Work out the finished part from the listing and answer in its coordinate system (mm). A direction names the side the tool comes from. Coordinates: 2 decimals unless noted, no trailing zeros. Order: outer loops, then holes, each group sorted by start corner. A loop starts at its lowest first (then second) coordinate and runs counter-clockwise, first axis right, second up. Notation, with made-up numbers: M 19.25,10.5 L 46.25,10.5 A21 cw 46.25,48.5 Z; hole C -12.75,78.5 d7. An arc over 180 degrees is marked long. Use a Markdown table: item, result. Add a question column.
from build123d import *

# Parameters (mm, degrees)
BOSS_EXTRUDE1_DEPTH      = 9.525
BOSS_EXTRUDE1_DEPTH_BACK = 9.525
SKETCH1_R                = 1.7
CUT_EXTRUDE1_DEPTH       = 6.35
CUT_EXTRUDE1_DEPTH_BACK  = 27.686
SKETCH2_W                = 2.54
SKETCH2_H                = 5.08
BOSS_EXTRUDE2_DEPTH      = 1.5875
BOSS_EXTRUDE3_START      = 1.5875
SKETCH5_R                = 1.7
BOSS_EXTRUDE3_DEPTH      = 1.5875
CUT_EXTRUDE2_START       = -5.08
CUT_EXTRUDE2_DEPTH       = 5.08
FILLET1_R                = 6.35
FILLET2_R                = 2.54
CHAMFER1_SIZE            = 0.5
SKETCH8_W                = 17.78
SKETCH8_H                = 50.8
CUT_EXTRUDE3_DEPTH       = 5.08
FILLET3_START            = -0.635
FILLET3_DEPTH            = 5.635


with BuildPart() as part:
    # Sketch1 → Boss-Extrude1 (new, two sides: drawn at the far end of the back side and taken through both)
    with BuildSketch(Plane.XY.offset(-BOSS_EXTRUDE1_DEPTH_BACK)):
        with BuildLine():
            Line((-107.95, 0), (-133.35, 0))
            Line((-133.35, 0), (-133.35, -17.78))
            Line((-133.35, -17.78), (-123.825, -17.78))
            ThreePointArc((-123.825, -17.78), (-117.475, -11.43), (-111.125, -17.78))
            Line((-111.125, -17.78), (-101.7905, -17.78))
            Line((-101.7905, -17.78), (-101.7905, -3.81))
            ThreePointArc((-101.7905, -3.81), (-100.302602448, -0.217897552), (-96.7105, 1.27))
            Line((-96.7105, 1.27), (-93.9165, 1.27))
            ThreePointArc((-93.9165, 1.27), (-90.324397552, -0.217897552), (-88.8365, -3.81))
            Line((-88.8365, -3.81), (-88.8365, -17.78))
            Line((-88.8365, -17.78), (-88.8365, -33.02))
            Line((-88.8365, -33.02), (88.8365, -33.02))
            Line((88.8365, -33.02), (88.8365, -17.78))
            Line((88.8365, -17.78), (88.8365, -3.81))
            ThreePointArc((88.8365, -3.81), (90.324397552, -0.217897552), (93.9165, 1.27))
            Line((93.9165, 1.27), (96.7105, 1.27))
            ThreePointArc((96.7105, 1.27), (100.302602448, -0.217897552), (101.7905, -3.81))
            Line((101.7905, -3.81), (101.7905, -17.78))
            Line((101.7905, -17.78), (111.125, -17.78))
            ThreePointArc((111.125, -17.78), (117.475, -11.43), (123.825, -17.78))
            Line((123.825, -17.78), (133.35, -17.78))
            Line((133.35, -17.78), (133.35, 0))
            Line((133.35, 0), (107.95, 0))
            Line((107.95, 0), (107.95, 17.78))
            Line((107.95, 17.78), (-107.95, 17.78))
            Line((-107.95, 17.78), (-107.95, 0))
        make_face()
        with Locations((-79.9465, -7.62)):
            Circle(SKETCH1_R, mode=Mode.SUBTRACT)
        with Locations((-79.9465, 11.43)):
            Circle(SKETCH1_R, mode=Mode.SUBTRACT)
        with Locations((79.9465, -7.62)):
            Circle(SKETCH1_R, mode=Mode.SUBTRACT)
        with Locations((79.9465, 11.43)):
            Circle(SKETCH1_R, mode=Mode.SUBTRACT)
    extrude(amount=BOSS_EXTRUDE1_DEPTH + BOSS_EXTRUDE1_DEPTH_BACK)

    # Sketch2 → Cut-Extrude1 (cut, two sides: drawn at the far end of the back side and taken through both)
    with BuildSketch(Plane(origin=(0, 0, 0), x_dir=(1, 0, 0), z_dir=(0, 1, 0)).offset(-CUT_EXTRUDE1_DEPTH_BACK)):
        with Locations((-106.68, 0)):
            Rectangle(SKETCH2_W, SKETCH2_H)
        with Locations((-132.08, 0)):
            Rectangle(SKETCH2_W, SKETCH2_H)
        with Locations((132.08, 0)):
            Rectangle(SKETCH2_W, SKETCH2_H)
        with Locations((106.68, 0)):
            Rectangle(SKETCH2_W, SKETCH2_H)
    extrude(amount=CUT_EXTRUDE1_DEPTH + CUT_EXTRUDE1_DEPTH_BACK, mode=Mode.SUBTRACT)

    # Sketch3 → Boss-Extrude2 (add)
    with BuildSketch(Plane.XY.offset(9.525)):
        with BuildLine():
            Line((-101.7905, -17.78), (-101.7905, 0))
            Line((-101.7905, 0), (-133.35, 0))
            Line((-133.35, 0), (-133.35, -17.78))
            Line((-133.35, -17.78), (-122.301, -17.78))
            ThreePointArc((-122.301, -17.78), (-117.475, -12.954), (-112.649, -17.78))
            Line((-112.649, -17.78), (-101.7905, -17.78))
        make_face()
        with BuildLine():
            Line((101.7905, -17.78), (112.649, -17.78))
            ThreePointArc((112.649, -17.78), (117.475, -12.954), (122.301, -17.78))
            Line((122.301, -17.78), (133.35, -17.78))
            Line((133.35, -17.78), (133.35, 0))
            Line((133.35, 0), (101.7905, 0))
            Line((101.7905, 0), (101.7905, -17.78))
        make_face()
    boss_extrude2 = extrude(amount=BOSS_EXTRUDE2_DEPTH)

    # Mirror1: Boss-Extrude2 across plane
    add(boss_extrude2.mirror(Plane.XY))

    # Sketch5 → Boss-Extrude3 (add)
    with BuildSketch(Plane(origin=(0, 0, -9.525), x_dir=(-1, 0, 0), z_dir=(0, 0, -1)).offset(BOSS_EXTRUDE3_START)):
        with BuildLine():
            Line((-107.95, 0), (-101.7905, 0))
            Line((-101.7905, 0), (-101.7905, -3.81))
            ThreePointArc((-101.7905, -3.81), (-100.302602448, -0.217897552), (-96.7105, 1.27))
            Line((-96.7105, 1.27), (-93.9165, 1.27))
            ThreePointArc((-93.9165, 1.27), (-90.324397552, -0.217897552), (-88.8365, -3.81))
            Line((-88.8365, -3.81), (-88.8365, -33.02))
            Line((-88.8365, -33.02), (88.8365, -33.02))
            Line((88.8365, -33.02), (88.8365, -3.81))
            ThreePointArc((88.8365, -3.81), (90.324397552, -0.217897552), (93.9165, 1.27))
            Line((93.9165, 1.27), (96.7105, 1.27))
            ThreePointArc((96.7105, 1.27), (100.302602448, -0.217897552), (101.7905, -3.81))
            Line((101.7905, -3.81), (101.7905, 0))
            Line((101.7905, 0), (107.95, 0))
            Line((107.95, 0), (107.95, 17.78))
            Line((107.95, 17.78), (-107.95, 17.78))
            Line((-107.95, 17.78), (-107.95, 0))
        make_face()
        with Locations(Location((-79.9465, -7.62, 0), (0, 0, 180))):
            Circle(SKETCH5_R, mode=Mode.SUBTRACT)
        with Locations(Location((-79.9465, 11.43, 0), (0, 0, 180))):
            Circle(SKETCH5_R, mode=Mode.SUBTRACT)
        with Locations(Location((79.9465, -7.62, 0), (0, 0, 180))):
            Circle(SKETCH5_R, mode=Mode.SUBTRACT)
        with Locations(Location((79.9465, 11.43, 0), (0, 0, 180))):
            Circle(SKETCH5_R, mode=Mode.SUBTRACT)
    extrude(amount=-BOSS_EXTRUDE3_DEPTH)

    # Sketch7 → Cut-Extrude2 (cut)
    with BuildSketch(Plane.XY.offset(9.525).offset(CUT_EXTRUDE2_START)):
        with BuildLine():
            Line((-88.8365, -33.02), (-88.8365, -3.81))
            ThreePointArc((-88.8365, -3.81), (-90.324397552, -0.217897552), (-93.9165, 1.27))
            Line((-93.9165, 1.27), (-96.7105, 1.27))
            ThreePointArc((-96.7105, 1.27), (-100.302602448, -0.217897552), (-101.7905, -3.81))
            Line((-101.7905, -3.81), (-101.7905, 0))
            Line((-101.7905, 0), (-107.95, 0))
            Line((-107.95, 0), (-107.95, 17.78))
            Line((-107.95, 17.78), (-71.0565, 17.78))
            Line((-71.0565, 17.78), (-71.0565, -33.02))
            Line((-71.0565, -33.02), (-88.8365, -33.02))
        make_face()
        with BuildLine():
            Line((71.0565, -33.02), (88.8365, -33.02))
            Line((88.8365, -33.02), (88.8365, -3.81))
            ThreePointArc((88.8365, -3.81), (90.324397552, -0.217897552), (93.9165, 1.27))
            Line((93.9165, 1.27), (96.7105, 1.27))
            ThreePointArc((96.7105, 1.27), (100.302602448, -0.217897552), (101.7905, -3.81))
            Line((101.7905, -3.81), (101.7905, 0))
            Line((101.7905, 0), (107.95, 0))
            Line((107.95, 0), (107.95, 17.78))
            Line((107.95, 17.78), (71.0565, 17.78))
            Line((71.0565, 17.78), (71.0565, -33.02))
        make_face()
    extrude(amount=CUT_EXTRUDE2_DEPTH, mode=Mode.SUBTRACT)

    # Fillet1
    fillet1_edges = [part.edges().sort_by_distance(p)[0] for p in [
        (-101.7905, -8.89, 11.1125),
        (101.7905, -8.89, 11.1125),
    ]]
    fillet(fillet1_edges, radius=FILLET1_R)

    # Fillet2
    fillet2_edges = [part.edges().sort_by_distance(p)[0] for p in [
        (105.41, 6.35, 0),
        (-105.41, 6.35, 0),
    ]]
    fillet(fillet2_edges, radius=FILLET2_R - 0.0001)  # a hair under: the kernel refuses the full size

    # Chamfer1
    chamfer1_edges = [part.edges().sort_by_distance(p)[0] for p in [
        (-107.21975, -17.78, -11.1125),
        (-117.475, -12.954, -11.1125),
        (-127.8255, -17.78, -11.1125),
        (-133.35, -8.89, -11.1125),
        (-101.7905, -10.795, -11.1125),
        (117.475, -12.954, -11.1125),
        (107.21975, -17.78, -11.1125),
        (120.65, 0, -11.1125),
        (133.35, -8.89, -11.1125),
        (127.8255, -17.78, -11.1125),
        (101.7905, -10.795, -11.1125),
        (-120.65, 0, -11.1125),
        (-81.6465, -7.62, -11.1125),
        (78.2465, 11.43, -11.1125),
        (78.2465, -7.62, -11.1125),
        (-81.6465, 11.43, -11.1125),
        (0, 17.78, -11.1125),
        (107.95, 8.89, -11.1125),
        (100.302602448, -0.217897552, -11.1125),
        (95.3135, 1.27, -11.1125),
        (90.324397552, -0.217897552, -11.1125),
        (88.8365, -18.415, -11.1125),
        (0, -33.02, -11.1125),
        (-88.8365, -18.415, -11.1125),
        (-90.324397552, -0.217897552, -11.1125),
        (-95.3135, 1.27, -11.1125),
        (-100.302602448, -0.217897552, -11.1125),
        (-107.95, 8.89, -11.1125),
    ]]
    chamfer(chamfer1_edges, length=CHAMFER1_SIZE)

    # Sketch8 → Cut-Extrude3 (cut)
    with BuildSketch(Plane.XY.offset(4.445)):
        with Locations((-79.9465, -7.62)):
            Rectangle(SKETCH8_W, SKETCH8_H)
        with Locations((79.9465, -7.62)):
            Rectangle(SKETCH8_W, SKETCH8_H)
    extrude(amount=-CUT_EXTRUDE3_DEPTH, mode=Mode.SUBTRACT)

    # Fillet3: read off the stored shape, not the designer's step
    # Fillet3 outline → Fillet3 (cut)
    with BuildSketch(Plane.XY.offset(FILLET3_START)):
        with BuildLine():
            ThreePointArc((92.223166667, 0.979469931), (89.910030316, 1.300303581), (88.8365, 3.374204897))
            Line((88.8365, 3.374204897), (88.8365, -3.81))
            ThreePointArc((88.8365, -3.81), (89.768697369, -0.877060633), (92.223166667, 0.979469931))
        make_face()
        with BuildLine():
            ThreePointArc((-88.8365, 3.374204897), (-89.910030316, 1.300303581), (-92.223166667, 0.979469931))
            ThreePointArc((-92.223166667, 0.979469931), (-89.768697369, -0.877060633), (-88.8365, -3.81))
            Line((-88.8365, -3.81), (-88.8365, 3.374204897))
        make_face()
    extrude(amount=FILLET3_DEPTH, mode=Mode.SUBTRACT)


solid = part.part
(1) A cutting plane is placed at A-A on y = -23. Write down the section's boundary in (x, z) (1 decimal), plus the area to 3 significant figures.
(2) Straight lines are drawn through the part: line 1 (X direction, y = -8, z = -8); line 2 (X direction, y = 11.43, z = -7.5); line 3 (X direction, y = -11, z = 1). For each, find the intervals that lie inside material, in ascending order.
(3) A cutting plane is placed at B-B on x = 25. Write down the section's boundary in (y, z) (1 decimal).
(4) Given P1, Ø12, axis at y = 9, z = -3, coming from the -X side; P2, Ø23.5, axis at x = -78, y = -19.5, coming from the +Z side (3 decimals); P3, Ø1.5, axis at y = -2.5, z = 0.5, coming from the -X side, each flat-ended and moving along its own axis, determine where each tip first touches the part or whether it passes through.
(5) The mould has two halves that part along Z. Classify faces 1 (the flat face through (-118, -12.7, -9.525)), 2 (the cylindrical face through (-117.581, -12.955, -10.061)), 3 (the conical face through (-117.58, -12.82, -10.75)): pulls with the +Z half, pulls with the -Z half, needs draft (parallel to the pull), parting line crosses it, or undercut.
(6) Which of the six approach directions +Z, -Z, +X, -X, +Y, -Y give full straight-line access (tool end or side, diameter ignored) to faces 4 (the flat face through (71.056, -8, 5)), 5 (the flat face through (-133.35, -9, -7)), 6 (the cylindrical face through (-90.285, -0.258, -4.862)), 7 (the conical face through (-90.265, -0.077, -10.755)), 8 (the cylindrical face through (-117.61, -11.43, -0.13))?
From the geometry:
| question | item | result |
|---|---|---|
| 1 | outline | M -88.8,-10.6 L -88.3,-11.1 L 88.3,-11.1 L 88.8,-10.6 L 88.8,-0.6 L 71.1,-0.6 L 71.1,9.5 L -71.1,9.5 L -71.1,-0.6 L -88.8,-0.6 Z |
| 1 | area | 3,310 mm2 |
| 2 | line 1 | x = -133.35 to -101.79, -88.84 to -81.6, -78.29 to 78.29, 81.6 to 88.84, 101.79 to 133.35 |
| 2 | line 2 | x = -107.95 to -81.65, -78.25 to 78.25, 81.65 to 107.95 |
| 2 | line 3 | x = -130.81 to -107.95, -105.41 to -101.79, -71.06 to 71.06, 101.79 to 105.41, 107.95 to 130.81 |
| 3 | outline | M -33,-10.6 L -32.5,-11.1 L 17.3,-11.1 L 17.8,-10.6 L 17.8,9.5 L -33,9.5 Z |
| 4 | P1 | stops at x = -107.95 |
| 4 | P2 | stops at z = 9.525 |
| 4 | P3 | stops at x = -130.81 |
| 5 | face 1 | undercut |
| 5 | face 2 | needs draft |
| 5 | face 3 | pulls with the -Z half |
| 6 | face 4 | +Z, +Y, -Y |
| 6 | face 5 | +Z, -Z, -X, +Y, -Y |
| 6 | face 6 | +Z, -Z, -Y |
| 6 | face 7 | -Z, -Y |
| 6 | face 8 | -Y |
